Read the model definition and answer for the solid it produces. Units are mm, in the model's axes. Round coordinates to 2 decimals unless told otherwise and drop trailing zeros. Loops run counter-clockwise (first coordinate to the right, second up) from the corner with the lowest first, then second, coordinate; pieces in that order, holes last. Notation, with made-up numbers: M 72,-39.5 L 79,-39.5 A35 cw 79,-2.5 Z; hole C 78.5,17.5 d8. An arc over 180 degrees is marked long. Write each question's results on one line, items separated by ' | '.
```python
from build123d import *

# Parameters (mm, degrees)
F0_R     = 10
F1_DEPTH = 10


with BuildPart() as f1:
    # F0 (on Top) → F1 (new body)
    with BuildSketch(Plane.XY):
        Polygon((-37.010255, 12.600002), (-19.689747, 12.600002), (-11.029493, 27.600002), (-19.689747, 42.600002), (-37.010255, 42.600002), (-45.670509, 27.600002), align=None)
        with Locations((-28.350001, 27.600002)):
            Circle(F0_R, mode=Mode.SUBTRACT)
    extrude(amount=-F1_DEPTH)


solid = f1.part
```
1. Determine the mould class of faces 1 (the face through (-28, 12.6, -5)), 2 (the face through (-19.1, 23.8, -4.9)), 3 (the face through (-15.3, 35, -4.9)) for opening direction Y: released by +Y, released by -Y, zero draft, split by the parting line, or undercut.
Completed:
face 1: released by -Y | face 2: undercut | face 3: released by +Y
2. Given P1, Ø6, axis at y = 17, z = -5.5, coming from the +X side; P2, Ø18, axis at x = -28.35, y = 27.6, coming from the -Z side; P3, Ø1, axis at y = 22, z = -5.5, coming from the -X side; P4, Ø6, axis at y = 37, z = -3.5, coming from the +X side, each flat-ended and moving along its own axis, determine where each tip first touches the part or whether it passes through.
Completed:
P1: stops at x = -15.42 | P2: passes through | P3: stops at x = -42.73 | P4: stops at x = -14.72
3. Find section B-B, the plane z = -5. Give the vertices of the cut face in (x, y), then the cut area to 3 significant figures.
Completed:
outline: M -45.67,27.6 L -37.01,12.6 L -19.69,12.6 L -11.03,27.6 L -19.69,42.6 L -37.01,42.6 Z; hole C -28.35,27.6 d20 | area: 465 mm2
4. Find section A-A, the plane x = -28.35. Give the vertices of the cut face in (y, z).
Completed:
outline: M 12.6,-10 L 17.6,-10 L 17.6,0 L 12.6,0 Z; M 37.6,-10 L 42.6,-10 L 42.6,0 L 37.6,0 Z
5. Find the intervals of material crossed by L1, parallel to Y at x = -28.35, z = -6; L2, parallel to X at y = 19, z = -8; L3, parallel to Y at x = -25, z = -9, in increasing order.
Completed:
L1: y = 12.6 to 17.6, 37.6 to 42.6 | L2: x = -40.71 to -33.45, -23.25 to -15.99 | L3: y = 12.6 to 18.18, 37.02 to 42.6
6. Find section C-C, the plane y = 25. Give the vertices of the cut face in (x, z), then the cut area to 3 significant figures.
Completed:
outline: M -44.17,-10 L -38.01,-10 L -38.01,0 L -44.17,0 Z; M -18.69,-10 L -12.53,-10 L -12.53,0 L -18.69,0 Z | area: 123 mm2
7. Find section D-D, the plane y = 17. Give the vertices of the cut face in (x, z), then the cut area to 3 significant figures.
Completed:
outline: M -39.55,-10 L -17.15,-10 L -17.15,0 L -39.55,0 Z | area: 224 mm2
